from build123d import *

# Parameters (mm, degrees)
F0_W     = 60
F0_H     = 60
F1_DEPTH = 1140
F2_R     = 8
F3_T     = -4


with BuildPart() as f1:
    # F0 (on Top) → F1 (new body)
    with BuildSketch(Plane.XY):
        Rectangle(F0_W, F0_H)
    extrude(amount=F1_DEPTH)

    # F2
    f2_edges = [f1.edges().sort_by_distance(p)[0] for p in [
        (-30, -30, 570),
        (-30, 30, 570),
        (30, -30, 570),
        (30, 30, 570),
    ]]
    fillet(f2_edges, radius=F2_R)

    # F3
    f3_openings = [f1.faces().sort_by_distance(p)[0] for p in [
        (0, 0, 1140),
        (0, 0, 0),
    ]]
    offset(amount=F3_T, openings=f3_openings)


solid = f1.part
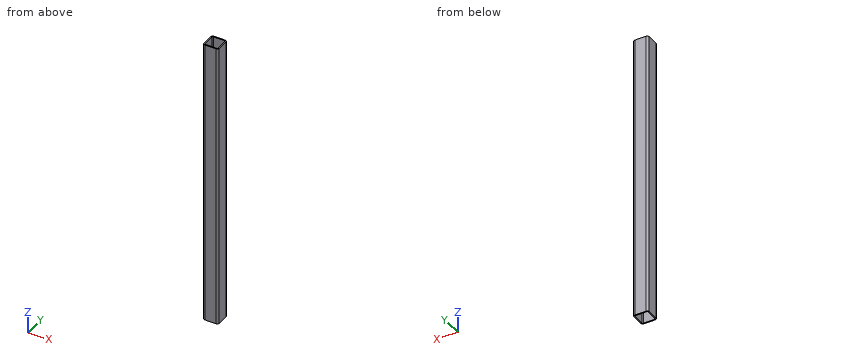
Source: CAD feature listing. Evaluate the final solid. Frame: model axes, mm. Round coordinates to 2 decimals unless told otherwise and drop trailing zeros. Order: outer loops, then holes, each group sorted by start corner. A loop starts at its lowest first (then second) coordinate and runs counter-clockwise, first axis right, second up. Notation, with made-up numbers: (87, -34) - (91, -34) arc R24 ccw to (91, -2) - close; hole circle Ø8 at (53, 83). An arc over 180 degrees is marked (long way). Use a Markdown table: item, result. Add a question column.
1. Line query: probe 1 along Y at (x, z) = (16, 76.5); probe 2 along Y at (x, z) = (23, 971). Output: solid intervals per line, ascending.
2. Section query A-A (y = -4.5). Return the cut outline in (x, z).
3. Section query C-C (z = 114.5). Return the cut outline in (x, y), then the cut area to 3 significant figures.
4. First-contact query: pin 1 (4 mm diameter, centred on x = -23.5, y = -6.5, fed in from -Z). Flat tip, straight axial feed; report the tip coordinate or a pass-through.
Derived:
| question | item | result |
|---|---|---|
| 1 | probe 1 | -30 to -26, 26 to 30 |
| 1 | probe 2 | -29.94 to -25.87, 25.87 to 29.94 |
| 2 | outline | (-30, 0) - (-26, 0) - (-26, 1140) - (-30, 1140) - close; (26, 0) - (30, 0) - (30, 1140) - (26, 1140) - close |
| 3 | outline | (-30, -22) arc R8 ccw to (-22, -30) - (22, -30) arc R8 ccw to (30, -22) - (30, 22) arc R8 ccw to (22, 30) - (-22, 30) arc R8 ccw to (-30, 22) - close; hole (-26, -22) arc R4 ccw to (-22, -26) - (22, -26) arc R4 ccw to (26, -22) - (26, 22) arc R4 ccw to (22, 26) - (-22, 26) arc R4 ccw to (-26, 22) - close |
| 3 | area | 855 mm2 |
| 4 | pin 1 | through |
